The model under review builds one solid part; all positions refer to its coordinate system, in mm. Face numbers are marked on the shaded views. A direction names the side the tool comes from. Give positions to 0.01 mm unless a question says otherwise; leave off trailing zeros. Order: outer loops, then holes, each group sorted by start corner. A loop starts at its lowest first (then second) coordinate and runs counter-clockwise, first axis right, second up. Notation, with made-up numbers: (36.25, 70.25) - (86.25, 70.25) arc R16 cw to (86.25, 85.25) - close; hole circle Ø10 at (0, 81). An arc over 180 degrees is marked (long way). Use CSV: the item, a comma, the result in double quotes. Start each with the question number.
1. Take a section at D-D, the plane z = 6.25. State the section outline as (x, y) points, then the cut area to 3 significant figures.
2. Take a section at B-B, the plane z = 17.75. State the section outline as (x, y) points.
3. To check wall thickness, follow line 1 (X direction, y = 0, z = 17); line 2 (X direction, y = 0, z = 7.5); line 3 (Y direction, x = 28, z = 5.25). State the ranges of each line that lie inside material, in increasing order. Write a range as [from, to].
4. For pin 1 (1 mm diameter, centred on y = 6.5, z = 14.5, fed in from +X); pin 2 (5 mm diameter, centred on x = 96.5, y = 10.5, fed in from -Z); pin 3 (4 mm diameter, centred on y = -6.5, z = 17.5, fed in from -X); pin 4 (3 mm diameter, centred on y = 12, z = 3.5, fed in from -X), all flat-tipped, find the tip position at first contact; note any pin that passes through.
5. Take a section at A-A, the plane y = 0. State the section outline as (x, z) points, then the cut area to 3 significant figures.
6. Take a section at C-C, the plane x = 66.5. State the section outline as (y, z) points, then the cut area to 3 significant figures.
7. Machinability: for the marked faces 5 and 6, which of the approach directions +Z, -Z, +X, -X, +Y, -Y give a long, thin tool a straight path to every point of the face, cutting with its end or side? Answer none if there is none.
8. Draft analysis for pull direction X (two halves, no side actions). For the marked faces 1, 2, 3 and 4, state which applies: released by +X, released by -X, zero draft, split by the parting line, or undercut.
Autodesk Inventor part; units mm, degrees
ref_plane "YZ Plane" through (0, 0, 0) normal (1, 0, 0) x (0, 1, 0)
ref_plane "XZ Plane" through (0, 0, 0) normal (0, 1, 0) x (-1, 0, 0)
ref_plane "XY Plane" through (0, 0, 0) normal (0, 0, 1) x (1, 0, 0)
sketch "Sketch1" plane through (0, 0, 0) normal (0, 0, 1) x (1, 0, 0)
  circle A0 centre (0, 0) radius 15
  circle A1 centre (127.2387, 0) radius 15
  line L0 (0, 15) -> (127.2387, 15)
  line L1 (0, -15) -> (127.2387, -15)
  line L2 (12.9904, -7.5) -> (114.2483, -7.5)
  line L3 (12.9904, 7.5) -> (114.2483, 7.5)
  dimension "d0" = 30
  dimension "d1" = 127.2387
  dimension "d2" = 7.5
  dimension "d3" = 7.5
extrude "Extrusion1" add sketch "Sketch1" along normal blind 20 contours A0 | A0 L0 A1 L3 | L2 A1 L1 A0 | A1
sketch "Sketch2" plane through (0, 0, 20) normal (0, 0, 1) x (1, 0, 0)
  arc A0 (127.2387, -15) -> (127.2387, 15) centre (127.2387, 0) ccw
  point P0 (0, 0)
  point P1 (142.2387, 0)
hole "Hole1" at (127.2387, 0, 20) direction (0, 0, -1) diameter 10 end through all counterbore diameter 22 counterbore depth 7
properties part number "PARALLEL_LINKAGE_LH"
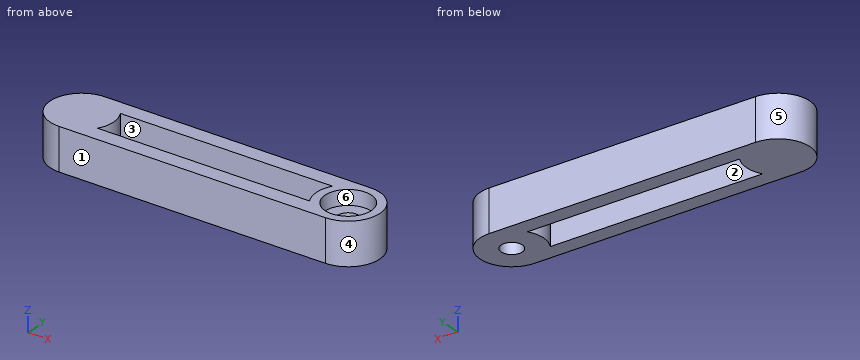
Determined:
1,outline,"(0, -15) - (127.24, -15) arc R15 ccw to (127.24, 15) - (0, 15) arc R15 ccw to start; hole (12.99, -7.5) - (114.25, -7.5) arc R15 cw to (114.25, 7.5) - (12.99, 7.5) arc R15 cw to start; hole circle Ø10 at (127.24, 0)"
1,area,"2,970 mm²"
2,outline,"(0, -15) - (127.24, -15) arc R15 ccw to (127.24, 15) - (0, 15) arc R15 ccw to start; hole (12.99, -7.5) - (114.25, -7.5) arc R15 cw to (114.25, 7.5) - (12.99, 7.5) arc R15 cw to start; hole circle Ø22 at (127.24, 0)"
3,line 1,"x = [-15, 15], [112.24, 116.24], [138.24, 142.24]"
3,line 2,"x = [-15, 15], [112.24, 122.24], [132.24, 142.24]"
3,line 3,"y = [-15, -7.5], [7.5, 15]"
4,pin 1,"stops at x = 140.99"
4,pin 2,"stops at z = 0"
4,pin 3,"stops at x = -14.31"
4,pin 4,"stops at x = -10.71"
5,outline,"(-15, 0) - (15, 0) - (15, 20) - (-15, 20) - close; (112.24, 0) - (122.24, 0) - (122.24, 13) - (116.24, 13) - (116.24, 20) - (112.24, 20) - close; (132.24, 0) - (142.24, 0) - (142.24, 20) - (138.24, 20) - (138.24, 13) - (132.24, 13) - close"
5,area,"916 mm²"
6,outline,"(-15, 0) - (-7.5, 0) - (-7.5, 20) - (-15, 20) - close; (7.5, 0) - (15, 0) - (15, 20) - (7.5, 20) - close"
6,area,"300 mm²"
7,face 5,"+Z, -Z, -X"
7,face 6,"+Z"
8,face 1,"zero draft"
8,face 2,"undercut"
8,face 3,"undercut"
8,face 4,"released by +X"
